from build123d import *

# Parameters (mm, degrees)
BOSS_EXTRUDE2_DEPTH = 9
CUT_EXTRUDE3_DEPTH  = 6
SKETCH5_R           = 1.5
CUT_EXTRUDE7_DEPTH  = 5
SKETCH7_R           = 1.5
CUT_EXTRUDE8_DEPTH  = 5
SKETCH8_R           = 1.5
CUT_EXTRUDE9_DEPTH  = 5


with BuildPart() as part:
    # Sketch1 → Boss-Extrude2 (new body)
    with BuildSketch(Plane(origin=(0, 0, 0), x_dir=(1, 0, 0), z_dir=(0, 1, 0))):
        Polygon((0, 51.961524227), (-45, 25.980762114), (-45, -25.980762114), (0, -51.961524227), (45, -25.980762114), (45, 25.980762114), align=None)
    extrude(amount=BOSS_EXTRUDE2_DEPTH)

    # Sketch4 → Cut-Extrude3 (cut)
    with BuildSketch(Plane.XZ):
        Polygon((0, 48.497422612), (-42, 24.248711306), (-42, -24.248711306), (0, -48.497422612), (42, -24.248711306), (42, 24.248711306), align=None)
    extrude(amount=-CUT_EXTRUDE3_DEPTH, mode=Mode.SUBTRACT)

    # Sketch5 → Cut-Extrude7 (cut)
    with BuildSketch(Plane.ZY.offset(45)):
        with Locations((-21.980762114, 3)):
            Circle(SKETCH5_R)
        with Locations((21.980762114, 3)):
            Circle(SKETCH5_R)
    extrude(amount=-CUT_EXTRUDE7_DEPTH, mode=Mode.SUBTRACT)

    # Sketch7 → Cut-Extrude8 (cut)
    with BuildSketch(Plane(origin=(22.5, 0, 38.97114317), x_dir=(0.8660254037844346, 0, -0.5000000000000071), z_dir=(0.5000000000000071, 0, 0.8660254037844346))):
        with Locations((-21.980762114, 3)):
            Circle(SKETCH7_R)
        with Locations((21.980762114, 3)):
            Circle(SKETCH7_R)
    extrude(amount=-CUT_EXTRUDE8_DEPTH, mode=Mode.SUBTRACT)

    # Sketch8 → Cut-Extrude9 (cut)
    with BuildSketch(Plane(origin=(22.5, 0, -38.97114317), x_dir=(-0.8660254037844414, 0, -0.49999999999999517), z_dir=(0.49999999999999517, 0, -0.8660254037844414))):
        with Locations((-21.980762114, 3)):
            Circle(SKETCH8_R)
        with Locations((21.980762114, 3)):
            Circle(SKETCH8_R)
    extrude(amount=-CUT_EXTRUDE9_DEPTH, mode=Mode.SUBTRACT)


solid = part.part
Work out the finished part from the listing and answer in its coordinate system (mm). A direction names the side the tool comes from. Coordinates: 2 decimals unless noted, no trailing zeros. Write each loop counter-clockwise with the first axis right and the second up, starting at its lowest first coordinate (ties: lowest second). Pieces come first, ordered by that corner, then holes. Notation, with made-up numbers: M 29,84.25 L 33,84.25 A35 cw 33,118.25 Z; hole C 28.25,78.25 d6. An arc over 180 degrees is marked long. Use one line per item in the form item = value. Start each with the question number.
1. Each of these flat-tipped pins is pushed along its axis until it touches: P1, Ø4, axis at x = -3, y = 6, coming from the -Z side; P2, Ø4, axis at x = 14.5, z = 16, coming from the -Y side; P3, Ø1.8, axis at y = 3, z = 21.98, coming from the -X side. Where does it stop, or does it pass through?
2. Straight lines are drawn through the part: probe 1 along X at (y, z) = (3.75, -10); probe 2 along Y at (x, z) = (-40.5, -23); probe 3 along X at (y, z) = (4.5, -43.5). For each, find the intervals that lie inside material, in ascending order. Write a range as from..to.
3. The part is cut by section C-C (x = -33.5). Give the vertices of the cut face in (y, z), plus the area to 3 significant figures.
4. The mould has two halves that part along Z. Classify faces 4 (the face through (-42, 3, 0)), 5 (the face through (-22.8, 4.4, 38.8)), 6 (the face through (-20, 0, 38)), 7 (the face through (-1, 6, 1)): released by +Z, released by -Z, zero draft, split by the parting line, or undercut.
5. The part is cut by section B-B (y = 7.5). Give the vertices of the cut face in (x, z).
6. A tool of negligible diameter and unlimited length cuts with its end or side. For faces 1 (the face through (42, 3, 0)), 2 (the face through (-45, 4, 0)), 3 (the face through (-43.52, 2.43, 23.37)), from which of +Z, -Z, +X, -X, +Y, -Y can it reach the whole face along a straight path? Write none if from no direction.
7. The part is cut by section A-A (z = 8.5). Give the vertices of the cut face in (x, y).
Evaluation:
q1.P1 = -51.38
q1.P2 = 6
q1.P3 = 42
q2.probe_1 = -45..-42, 42..45
q2.probe_2 = 6..9
q2.probe_3 = -14.66..-8.66, 8.66..14.66
q3.outline = M 0,-32.62 L 9,-32.62 L 9,32.62 L 0,32.62 L 0,29.16 L 6,29.16 L 6,-29.16 L 0,-29.16 Z
q3.area = 237 mm^2
q4.face_4 = undercut
q4.face_5 = released by +Z
q4.face_6 = zero draft
q4.face_7 = undercut
q5.outline = M -45,-25.98 L 0,-51.96 L 45,-25.98 L 45,25.98 L 0,51.96 L -45,25.98 Z
q6.face_1 = -Y
q6.face_2 = +Z, -Z, -X, +Y, -Y
q6.face_3 = -X
q7.outline = M -45,0 L -42,0 L -42,6 L 42,6 L 42,0 L 45,0 L 45,9 L -45,9 Z
